Source: CAD feature listing. Evaluate the final solid. Frame: model axes, mm. A direction names the side the tool comes from. Coordinates: 2 decimals unless noted, no trailing zeros. Order: outer loops, then holes, each group sorted by start corner. A loop starts at its lowest first (then second) coordinate and runs counter-clockwise, first axis right, second up.
Item 1: Section C-C on y = -7. Return the cut outline in (x, z), then the cut area to 4 significant figures.
Item 2: Section B-B on x = 8.5. Return the cut outline in (y, z).
Item 3: Reachability of faces 1 (the flat face through (-32.215, 0, 3)), 2 (the flat face through (-3, 11.5, 3)), 3 (the flat face through (19, 15, 3)), 4 (the flat face through (20, 6.4, 3)) from +Z, -Z, +X, -X, +Y, -Y: full face, straight path, thin tool, end or side. Return the list, or none.
Item 4: Section A-A on y = 0. Return the cut outline in (x, z).
Item 5: Ray query, line 1 (Y direction, x = 19.15, z = 2.15); line 2 (X direction, y = -8.5, z = 3.75); line 3 (Y direction, x = -9.5, z = 1.75). Return the intervals inside material, ascending.
Item 6: Section D-D on z = 1. State how many separate pieces and enclosed holes the cut face has, then the cut area to 3 significant figures.
Item 7: Mould query, pull axis Y, two halves, no side actions, for faces 5 (the cylindrical face through (-31.93, -3.35, 3.45)), 6 (the flat face through (-21, 6.4, 4)), 7 (the flat face through (17.15, 16, 3)). Classes: released by +Y, released by -Y, zero draft, split by the parting line, or undercut.
Item 8: Contact query for flat-ended pins moving along their axis: P1, Ø3.5, axis at y = 7.5, z = 3, coming from the -X side; P2, Ø3.5, axis at x = 19.15, y = -14.97, coming from the -Z side; P3, Ø3, axis at x = -29, z = 3.5, coming from the -Y side. Output: stop coordinate, or through.
from build123d import *

# Parameters (mm, degrees)
CROQUIS1_R              = 1.55
SALIENTE_EXTRUIR1_DEPTH = 5.5
CROQUIS2_R              = 1.55
SALIENTE_EXTRUIR2_DEPTH = 1.5
CROQUIS3_W              = 43.5
CROQUIS3_H              = 19
CORTAR_EXTRUIR1_DEPTH   = 1.9
CROQUIS4_R              = 1.5
CORTAR_EXTRUIR2_DEPTH   = 3
CHAFL_N1_SIZE           = 0.4


with BuildPart() as part:
    # Croquis1 → Saliente-Extruir1 (new body)
    with BuildSketch(Plane.XY):
        with BuildLine():
            Line((16.15, 11.5), (-23.25, 11.5))
            ThreePointArc((-23.25, 11.5), (-23.957106781, 11.207106781), (-24.25, 10.5))
            Line((-24.25, 10.5), (-24.25, 4.65))
            ThreePointArc((-24.25, 4.65), (-24.542893219, 3.942893219), (-25.25, 3.65))
            Line((-25.25, 3.65), (-31.215212315, 3.65))
            ThreePointArc((-31.215212315, 3.65), (-31.922319096, 3.357106781), (-32.215212315, 2.65))
            Line((-32.215212315, 2.65), (-32.215212315, -2.65))
            ThreePointArc((-32.215212315, -2.65), (-31.922319096, -3.357106781), (-31.215212315, -3.65))
            Line((-31.215212315, -3.65), (-25.25, -3.65))
            ThreePointArc((-25.25, -3.65), (-24.542893219, -3.942893219), (-24.25, -4.65))
            Line((-24.25, -4.65), (-24.25, -10.5))
            ThreePointArc((-24.25, -10.5), (-23.957106781, -11.207106781), (-23.25, -11.5))
            Line((-23.25, -11.5), (16.15, -11.5))
            ThreePointArc((16.15, -11.5), (16.857106781, -11.792893219), (17.15, -12.5))
            Line((17.15, -12.5), (17.15, -18.465212315))
            ThreePointArc((17.15, -18.465212315), (17.442893219, -19.172319096), (18.15, -19.465212315))
            Line((18.15, -19.465212315), (21.15, -19.465212315))
            Line((21.15, -19.465212315), (21.15, -6.4))
            Line((21.15, -6.4), (19.5, -6.4))
            Line((19.5, -6.4), (19.5, -9.5))
            Line((19.5, -9.5), (-19.5, -9.5))
            Line((-19.5, -9.5), (-19.5, -6.4))
            Line((-19.5, -6.4), (-22.5, -6.4))
            Line((-22.5, -6.4), (-22.5, 6.4))
            Line((-22.5, 6.4), (-19.5, 6.4))
            Line((-19.5, 6.4), (-19.5, 9.5))
            Line((-19.5, 9.5), (19.5, 9.5))
            Line((19.5, 9.5), (19.5, 6.4))
            Line((19.5, 6.4), (21.15, 6.4))
            Line((21.15, 6.4), (21.15, 19.465212315))
            Line((21.15, 19.465212315), (18.15, 19.465212315))
            ThreePointArc((18.15, 19.465212315), (17.442893219, 19.172319096), (17.15, 18.465212315))
            Line((17.15, 18.465212315), (17.15, 12.5))
            ThreePointArc((17.15, 12.5), (16.857106781, 11.792893219), (16.15, 11.5))
        make_face()
        with Locations((-28.232606158, 0)):
            Circle(CROQUIS1_R, mode=Mode.SUBTRACT)
    extrude(amount=SALIENTE_EXTRUIR1_DEPTH)

    # Croquis2 → Saliente-Extruir2 (add)
    with BuildSketch(Plane.XY.offset(5.5)):
        with BuildLine():
            Line((21.15, -6.4), (21.15, 6.4))
            Line((21.15, 6.4), (21.15, 19.465212315))
            Line((21.15, 19.465212315), (18.15, 19.465212315))
            ThreePointArc((18.15, 19.465212315), (17.442893219, 19.172319096), (17.15, 18.465212315))
            Line((17.15, 18.465212315), (17.15, 12.5))
            ThreePointArc((17.15, 12.5), (16.857106781, 11.792893219), (16.15, 11.5))
            Line((16.15, 11.5), (-23.25, 11.5))
            ThreePointArc((-23.25, 11.5), (-23.957106781, 11.207106781), (-24.25, 10.5))
            Line((-24.25, 10.5), (-24.25, 4.65))
            ThreePointArc((-24.25, 4.65), (-24.542893219, 3.942893219), (-25.25, 3.65))
            Line((-25.25, 3.65), (-31.215212315, 3.65))
            ThreePointArc((-31.215212315, 3.65), (-31.922319096, 3.357106781), (-32.215212315, 2.65))
            Line((-32.215212315, 2.65), (-32.215212315, -2.65))
            ThreePointArc((-32.215212315, -2.65), (-31.922319096, -3.357106781), (-31.215212315, -3.65))
            Line((-31.215212315, -3.65), (-25.25, -3.65))
            ThreePointArc((-25.25, -3.65), (-24.542893219, -3.942893219), (-24.25, -4.65))
            Line((-24.25, -4.65), (-24.25, -10.5))
            ThreePointArc((-24.25, -10.5), (-23.957106781, -11.207106781), (-23.25, -11.5))
            Line((-23.25, -11.5), (16.15, -11.5))
            ThreePointArc((16.15, -11.5), (16.857106781, -11.792893219), (17.15, -12.5))
            Line((17.15, -12.5), (17.15, -18.465212315))
            ThreePointArc((17.15, -18.465212315), (17.442893219, -19.172319096), (18.15, -19.465212315))
            Line((18.15, -19.465212315), (21.15, -19.465212315))
            Line((21.15, -19.465212315), (21.15, -6.4))
        make_face()
        with Locations((-28.232606158, 0)):
            Circle(CROQUIS2_R, mode=Mode.SUBTRACT)
    extrude(amount=SALIENTE_EXTRUIR2_DEPTH)

    # Croquis3 → Cortar-Extruir1 (cut)
    with BuildSketch(Plane(origin=(0, 0, 0), x_dir=(-1, 0, 0), z_dir=(0, 0, -1))):
        with Locations((0.75, 0)):
            Rectangle(CROQUIS3_W, CROQUIS3_H)
    extrude(amount=-CORTAR_EXTRUIR1_DEPTH, mode=Mode.SUBTRACT)

    # Croquis4 → Cortar-Extruir2 (cut)
    with BuildSketch(Plane(origin=(0, 0, 0), x_dir=(-1, 0, 0), z_dir=(0, 0, -1))):
        with Locations((-19.15, -14.965212315)):
            Circle(CROQUIS4_R)
        with Locations((-19.15, 14.965212315)):
            Circle(CROQUIS4_R)
    extrude(amount=-CORTAR_EXTRUIR2_DEPTH, mode=Mode.SUBTRACT)

    # Chaflán1
    chafl_n1_edges = [part.edges().sort_by_distance(p)[0] for p in [
        (20.65, -14.965212315, 0),
        (20.65, 14.965212315, 0),
    ]]
    chamfer(chafl_n1_edges, length=CHAFL_N1_SIZE)


solid = part.part
Answer list:
1. outline: (-24.25, 0) - (-22.5, 0) - (-22.5, 1.9) - (-19.5, 1.9) - (-19.5, 5.5) - (19.5, 5.5) - (19.5, 1.9) - (21, 1.9) - (21, 0) - (21.15, 0) - (21.15, 7) - (-24.25, 7) - close
1. area: 94.75 mm2
2. outline: (-11.5, 0) - (-9.5, 0) - (-9.5, 5.5) - (9.5, 5.5) - (9.5, 0) - (11.5, 0) - (11.5, 7) - (-11.5, 7) - close
3. face 1: +Z, -Z, -X, +Y, -Y
3. face 2: +Z, -Z, -X, +Y
3. face 3: -Z
3. face 4: -Z, +X
4. outline: (-32.22, 0) - (-29.78, 0) - (-29.78, 7) - (-32.22, 7) - close; (-26.68, 0) - (-22.5, 0) - (-22.5, 5.5) - (21.15, 5.5) - (21.15, 7) - (-26.68, 7) - close
5. line 1: y = -19.47 to -16.47, -13.47 to -9.5, 9.5 to 13.47, 16.47 to 19.47
5. line 2: x = -24.25 to -19.5, 19.5 to 21.15
5. line 3: y = -11.5 to -9.5, 9.5 to 11.5
6. separate pieces: 1
6. enclosed holes: 3
6. area: 316 mm2
7. face 5: released by -Y
7. face 6: undercut
7. face 7: zero draft
8. P1: stops at x = -24.25
8. P2: stops at z = 0.15
8. P3: stops at y = -3.65
